from build123d import *

# Parameters (mm, degrees)
M3_TAPPED_HOLE1_REACH  = 23.2
M3_TAPPED_HOLE1_BORE_R = 1.25
CUT_EXTRUDE1_DEPTH     = 7
CIRPATTERN1_COUNT      = 20


with BuildPart() as part:
    # Sketch1 → Revolve1 (revolve)
    with BuildSketch(Plane.XY, mode=Mode.PRIVATE) as revolve1_sk:
        Polygon((0, 2.5), (15.2, 2.5), (15.2, 8.05), (13.1, 8.05), (13.1, 6.365), (6.1, 6.365), (6.1, 8.05), (0, 8.05), align=None)
    revolve(revolve1_sk.sketch.rotate(Axis((0, 0, 0), (1, 0, 0)), 90), axis=Axis((0, 0, 0), (1, 0, 0)))

    # M3 Tapped Hole1 bore (on position points) → M3 Tapped Hole1 (cut, up to next)
    with BuildSketch(Plane(origin=(4, 8.05, 0), x_dir=(0, 0, 1), z_dir=(0, 1, 0)), mode=Mode.PRIVATE) as m3_tapped_hole1_sk1:
        Circle(M3_TAPPED_HOLE1_BORE_R)
    m3_tapped_hole1_tool1 = extrude(m3_tapped_hole1_sk1.sketch, amount=-M3_TAPPED_HOLE1_REACH, mode=Mode.PRIVATE) & part.part
    add(m3_tapped_hole1_tool1.solids().sort_by_distance((4, 8.05, 0))[0], mode=Mode.SUBTRACT)

    # Sketch3 → Cut-Extrude1 (cut)
    with BuildSketch(Plane.ZY.offset(-13.1)):
        Polygon((-0.6, 6.365), (-0.308823813, 5.565), (0.308823813, 5.565), (0.6, 6.365), align=None)
    cut_extrude1 = extrude(amount=CUT_EXTRUDE1_DEPTH, mode=Mode.SUBTRACT)

    # CirPattern1: Cut-Extrude1 ×20 about axis
    cirpattern1_axis = Axis((0, 0, 0), (1, 0, 0))
    for i in range(1, CIRPATTERN1_COUNT):
        add(cut_extrude1.rotate(cirpattern1_axis, i * 360 / CIRPATTERN1_COUNT), mode=Mode.SUBTRACT)


solid = part.part
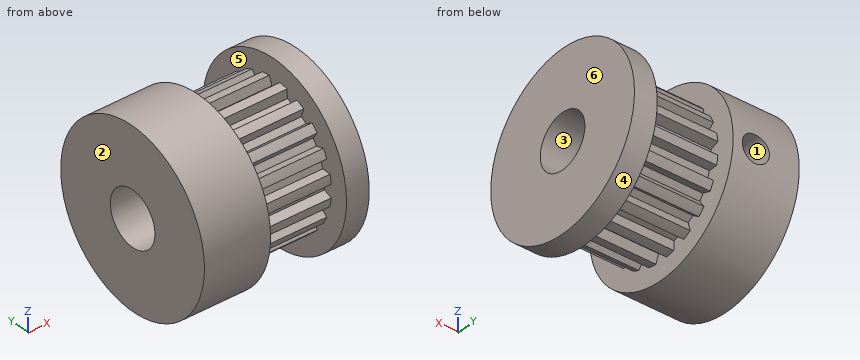
The listing builds one solid part. Answer for the finished solid, in the listing's coordinates (mm). Face numbers are marked on the shaded views. A direction names the side the tool comes from. Round coordinates to 2 decimals unless told otherwise and drop trailing zeros. Write each loop counter-clockwise with the first axis right and the second up, starting at its lowest first coordinate (ties: lowest second). Pieces come first, ordered by that corner, then holes. Notation, with made-up numbers: (0, 89) - (11, 89) arc R13 cw to (11, 110) - close; hole circle Ø9 at (84.5, 58). An arc over 180 degrees is marked (long way). Use one line per item in the form item = value. Start each with the question number.
Item 1: Find the intervals of material crossed by line 1 (X direction, y = 5, z = 0); line 2 (X direction, y = 6.1, z = 0); line 3 (X direction, y = -0.75, z = 7.25), in increasing order. Write a range as [from, to].
Item 2: Flat-ended cylindrical pins translate along their axes: pin 1 Ø8 at (x, y) = (5, 5) entering from +Z; pin 2 Ø1.5 at (x, y) = (11.5, 4.5) entering from +Z; pin 3 Ø1.5 at (x, y) = (3.5, 1) entering from -Z; pin 4 Ø4.5 at (y, z) = (0, 0) entering from -X. Find the tip coordinate at first contact, or state that the pin passes through.
Item 3: A cutting plane is placed at B-B (z = 0). Write down the section's boundary in (x, y) (3 decimals), plus the area to 3 significant figures.
Item 4: A cutting plane is placed at C-C (x = 2). Write down the section's boundary in (y, z), plus the area to 3 significant figures.
Item 5: A tool of negligible diameter and unlimited length cuts with its end or side. For the marked faces 5 and 6, from which of +Z, -Z, +X, -X, +Y, -Y can it reach the whole face along a straight path? Write none if from no direction.
Item 6: A cutting plane is placed at A-A (y = 0). Write down the section's boundary in (x, z) (3 decimals), plus the area to 3 significant figures.
Item 7: Determine the mould class of the marked faces 1, 2, 3 and 4 for opening direction Z: +Z half, -Z half, draft (parallel to the pull), parting line (faces both ways), or undercut.
Item 8: A cutting plane is placed at D-D (y = -2.25). Write down the section's boundary in (x, z), plus the area to 3 significant figures.
The answers:
q1.line_1 = [0, 2.75], [5.25, 15.2]
q1.line_2 = [0, 2.75], [5.25, 6.1], [13.1, 15.2]
q1.line_3 = [0, 6.1], [13.1, 15.2]
q2.pin_1 = 7.99
q2.pin_2 = 4.78
q2.pin_3 = -8.05
q2.pin_4 = through
q3.outline = (0, -8.05) - (6.1, -8.05) - (6.1, -5.565) - (13.1, -5.565) - (13.1, -8.05) - (15.2, -8.05) - (15.2, -2.5) - (0, -2.5) - close; (0, 2.5) - (2.75, 2.5) - (2.75, 8.05) - (0, 8.05) - close; (5.25, 2.5) - (15.2, 2.5) - (15.2, 8.05) - (13.1, 8.05) - (13.1, 5.565) - (6.1, 5.565) - (6.1, 8.05) - (5.25, 8.05) - close
q3.area = 120 mm^2
q4.outline = circle Ø16.1 at (0, 0); hole circle Ø5 at (0, 0)
q4.area = 184 mm^2
q5.face_5 = none
q5.face_6 = +Z, -Z, +X, +Y, -Y
q6.outline = (0, -8.05) - (6.1, -8.05) - (6.1, -5.565) - (13.1, -5.565) - (13.1, -8.05) - (15.2, -8.05) - (15.2, -2.5) - (0, -2.5) - close; (0, 2.5) - (15.2, 2.5) - (15.2, 8.05) - (13.1, 8.05) - (13.1, 5.565) - (6.1, 5.565) - (6.1, 8.05) - (0, 8.05) - close
q6.area = 134 mm^2
q7.face_1 = undercut
q7.face_2 = draft
q7.face_3 = undercut
q7.face_4 = parting line
q8.outline = (0, -7.73) - (6.1, -7.73) - (6.1, -5.5) - (13.1, -5.5) - (13.1, -7.73) - (15.2, -7.73) - (15.2, -1.09) - (0, -1.09) - close; (0, 1.09) - (15.2, 1.09) - (15.2, 7.73) - (13.1, 7.73) - (13.1, 5.5) - (6.1, 5.5) - (6.1, 7.73) - (0, 7.73) - close
q8.area = 171 mm^2
